CAD build for the part. Positions are in the model's coordinates, mm. Face numbers are marked on the shaded views. Coordinates: 2 decimals unless noted, no trailing zeros. Order: outer loops, then holes, each group sorted by start corner. A loop starts at its lowest first (then second) coordinate and runs counter-clockwise, first axis right, second up. Notation, with made-up numbers: M 21,7 L 52,7 A17 cw 52,40 Z; hole C -9,-15 d11. An arc over 180 degrees is marked long. Write item = value, one per line.
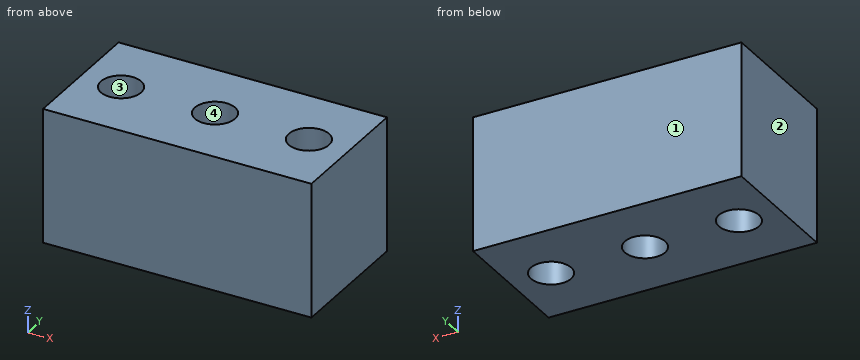
Autodesk Inventor part; units mm, degrees
ref_plane "YZ Plane" through (0, 0, 0) normal (1, 0, 0) x (0, 1, 0)
ref_plane "XZ Plane" through (0, 0, 0) normal (0, 1, 0) x (-1, 0, 0)
ref_plane "XY Plane" through (0, 0, 0) normal (0, 0, 1) x (1, 0, 0)
sketch "スケッチ1" plane through (0, 0, 0) normal (0, 0, 1) x (1, 0, 0)
  line L0 (0, 0) -> (20, 0)
  line L1 (20, 0) -> (20, 10)
  line L2 (20, 10) -> (0, 10)
  line L3 (0, 10) -> (0, 0)
  dimension "d0" = 20
  dimension "d1" = 10
extrude "押し出し1" add sketch "スケッチ1" along normal blind 10
sketch "スケッチ3" plane through (0, 0, 10) normal (0, 0, 1) x (1, 0, 0)
  line L0 (20, 10) -> (0, 10)
  point P0 (0, 0)
  point P1 (10, 5)
  dimension "d13" = 5
hole "穴2" at (10, 5, 10) direction (0, 0, -1) diameter 3 end through all
sketch "スケッチ4" plane through (0, 0, 10) normal (0, 0, 1) x (1, 0, 0)
  line L0 (0, 10) -> (0, 0)
  line L1 (20, 0) -> (20, 10)
  point P0 (3, 5)
  point P1 (17, 5)
  dimension "d21" = 3
  dimension "d22" = 3
hole "穴3" at (3, 5, 10) at (17, 5, 10) direction (0, 0, -1) diameter 3 end through all
properties part number "指下"
(1) Pull direction X, two halves, no side cores. Call the marked faces 1, 2, 3 and 4: +X half, -X half, draft (parallel to the pull), parting line (faces both ways), or undercut.
Evaluation:
face_1 = draft
face_2 = -X half
face_3 = undercut
face_4 = undercut
(2) Slice it at A-A, the plane z = 0.5. Write the cut outline in (x, y).
Evaluation:
outline = M 0,0 L 20,0 L 20,10 L 0,10 Z; hole C 3,5 d3; hole C 10,5 d3; hole C 17,5 d3
(3) Slice it at C-C, the plane x = 3. Write the cut outline in (y, z), then the cut area to 3 significant figures.
Evaluation:
outline = M 0,0 L 3.5,0 L 3.5,10 L 0,10 Z; M 6.5,0 L 10,0 L 10,10 L 6.5,10 Z
area = 70.0 mm²
(4) Wall check: line 1 (X direction, y = 5, z = 7); line 2 (X direction, y = 4, z = 3.25); line 3 (Y direction, x = 17, z = 2.5). Give the ranges that are in metal, low to high. Write a range as from..to.
Evaluation:
line_1 = 0..1.5, 4.5..8.5, 11.5..15.5, 18.5..20
line_2 = 0..1.88, 4.12..8.88, 11.12..15.88, 18.12..20
line_3 = 0..3.5, 6.5..10
(5) Slice it at B-B, the plane y = 5. Write the cut outline in (x, z).
Evaluation:
outline = M 0,0 L 1.5,0 L 1.5,10 L 0,10 Z; M 4.5,0 L 8.5,0 L 8.5,10 L 4.5,10 Z; M 11.5,0 L 15.5,0 L 15.5,10 L 11.5,10 Z; M 18.5,0 L 20,0 L 20,10 L 18.5,10 Z
